from build123d import *

# Parameters (mm, degrees)
BOSS_EXTRUDE1_DEPTH     = 6.35
CHAMFER1_SIZE           = 2.032
F_1_4_CLEARANCE_HOLE1_D = 6.7564
LPATTERN1_COUNT         = 4
LPATTERN1_PITCH         = 63.5


with BuildPart() as part:
    # Sketch1 → Boss-Extrude1 (new body)
    with BuildSketch(Plane.XY):
        Polygon((101.6, 12.7), (101.6, -76.2), (95.25, -76.2), (0, -38.1), (-25.4, -38.1), (-25.4, 0), (-25.4, 228.6), (0, 228.6), align=None)
    extrude(amount=BOSS_EXTRUDE1_DEPTH)

    # Chamfer1
    chamfer1_edges = [part.edges().sort_by_distance(p)[0] for p in [
        (50.8, 120.65, 0),
        (50.8, 120.65, 6.35),
    ]]
    chamfer(chamfer1_edges, length=CHAMFER1_SIZE)

    # 1/4 Clearance Hole1 (through all)
    with Locations(Plane.XY.offset(6.35)):
        with Locations((-10.31875, 203.2)):
            f_1_4_clearance_hole1 = Hole(F_1_4_CLEARANCE_HOLE1_D / 2)

    # LPattern1: 1/4 Clearance Hole1 ×4
    with Locations(*[(0, -i * LPATTERN1_PITCH, 0) for i in range(1, LPATTERN1_COUNT)]):
        add(f_1_4_clearance_hole1, mode=Mode.SUBTRACT)


solid = part.part
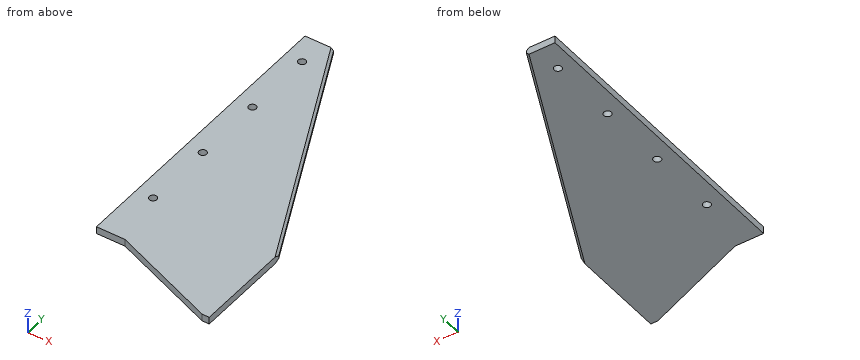
Design review of the part built by this model. Coordinates are the model's own, in mm. Round coordinates to 2 decimals unless told otherwise and drop trailing zeros. Write each loop counter-clockwise with the first axis right and the second up, starting at its lowest first coordinate (ties: lowest second). Pieces come first, ordered by that corner, then holes. Notation, with made-up numbers: (73, -13) -> (96, -13) arc R25 cw to (96, 13) -> close; hole circle Ø10 at (5, -30). An arc over 180 degrees is marked (long way). One line per question, with ' | ' between items.
(1) Take a section at B-B, the plane y = 139.7. State the section outline as (x, z) points, and give its area (3 significant figures).
Result sheet:
outline: (-25.4, 0) -> (-13.7, 0) -> (-13.7, 6.35) -> (-25.4, 6.35) -> close; (-6.94, 0) -> (39.59, 0) -> (41.84, 2.03) -> (41.84, 4.32) -> (39.59, 6.35) -> (-6.94, 6.35) -> close | area: 379 mm2
(2) Insertion check: P1, Ø1, axis at y = 175.5, z = 3, coming from the +X side; P2, Ø3, axis at x = 50, z = 5, coming from the +Y side; P3, Ø3, axis at x = -10, z = 4, coming from the -Y side. Each pin has a flat end and moves straight along its axis. Give the tip position at first contact, or say it passes through.
Result sheet:
P1: x = 25.22 | P2: y = 125.19 | P3: y = -38.1
(3) Take a section at D-D, the plane x = 91. State the section outline as (y, z) points (3 decimals).
Result sheet:
outline: (-74.5, 0) -> (30.453, 0) -> (35.225, 2.032) -> (35.225, 4.318) -> (30.453, 6.35) -> (-74.5, 6.35) -> close
(4) Take a section at C-C, the plane y = -49.5. State the section outline as (x, z) points.
Result sheet:
outline: (28.5, 0) -> (101.6, 0) -> (101.6, 6.35) -> (28.5, 6.35) -> close
(5) Take a section at A-A, the plane z = 3. State the section outline as (x, y) points.
Result sheet:
outline: (-25.4, -38.1) -> (0, -38.1) -> (95.25, -76.2) -> (101.6, -76.2) -> (101.6, 12.7) -> (0, 228.6) -> (-25.4, 228.6) -> close; hole circle Ø6.76 at (-10.32, 12.7); hole circle Ø6.76 at (-10.32, 76.2); hole circle Ø6.76 at (-10.32, 139.7); hole circle Ø6.76 at (-10.32, 203.2)
(6) Wall thickness on line 1 (X direction, y = 139.7, z = 2.25); line 2 (X direction, y = 203.2, z = 4); line 3 (Y direction, x = -17, z = 5): over which ranges is each line inside the solid? List them lowest first. Write a range as [from, to].
Result sheet:
line 1: [-25.4, -13.7], [-6.94, 41.84] | line 2: [-25.4, -13.7], [-6.94, 11.95] | line 3: [-38.1, 228.6]
